Build history of the part. All positions in model axes, mm. Face numbers are marked on the shaded views. A direction names the side the tool comes from. Give positions to 0.01 mm unless a question says otherwise; leave off trailing zeros. Order: outer loops, then holes, each group sorted by start corner. A loop starts at its lowest first (then second) coordinate and runs counter-clockwise, first axis right, second up. Notation, with made-up numbers: (88, 70) -> (128, 70) arc R22 ccw to (128, 96) -> close; hole circle Ø2 at (31, 77). An arc over 180 degrees is marked (long way). One line per question, with ' | ' between items. Start each with the question number.
(1) Cut at A-A (y = 4). Give the cut face in (x, z) (3 decimals).
(2) Pin check, flat tips, straight feed: pin 1 Ø2.5 at (x, z) = (22.5, -14.5) entering from -Y (3 decimals); pin 2 Ø4 at (x, z) = (14, -29) entering from +Y (3 decimals); pin 3 Ø1.9 at (y, z) = (4, -10) entering from -X; pin 4 Ø1.5 at (x, z) = (-4, -19) entering from +Y. Stop position of each tip, or through.
(3) Drill centre lines: L1, parallel to X at y = 3.5, z = -11.43; L2, parallel to Z at x = 8, y = 2.25; L3, parallel to X at y = 1, z = -11.5. Where is each one in solid material? Low to high. Write a range as from..to.
(4) Which spindle directions (+Z, -Z, +X, -X, +Y, -Y) get a long thin tool onto all of the face, cutting with end or side? Do the marked faces 1, 2, 3 and 4. Say none if no direction does.
(5) Cut at C-C (z = -12.7). Give the cut face in (x, y) (3 decimals), then the cut area to 3 significant figures.
(6) Cut at D-D (y = 0.5). Give the cut face in (x, z) (3 decimals).
(7) Cut at B-B (x = 12.7). Give the cut face in (y, z) (3 decimals).
Autodesk Inventor part; units mm, degrees
ref_plane "YZ Plane" through (0, 0, 0) normal (1, 0, 0) x (0, 1, 0)
ref_plane "XZ Plane" through (0, 0, 0) normal (0, 1, 0) x (-1, 0, 0)
ref_plane "XY Plane" through (0, 0, 0) normal (0, 0, 1) x (1, 0, 0)
sketch "Sketch1" plane through (0, 0, 0) normal (0, 1, 0) x (-1, 0, 0)
  line L0 (0, 0) -> (-25.4, 0)
  line L1 (-25.4, 0) -> (-25.4, -25.4)
  line L2 (-25.4, -25.4) -> (0, -25.4)
  line L3 (0, -25.4) -> (0, 0)
  dimension "d0" = 25.4
extrude "Extrusion1" add sketch "Sketch1" along normal blind 6.35
sketch "Sketch2" plane through (0, 6.35, 0) normal (0, 1, 0) x (1, 0, 0)
  circle A0 centre (8.4667, 13.97) radius 0.635
  circle A1 centre (16.9333, 13.97) radius 0.635
  circle A2 centre (16.9333, 11.43) radius 0.635
  circle A3 centre (8.4667, 11.43) radius 0.635
  line L0 (25.4, 0) -> (25.4, 25.4)
  line L1 (0, 0) -> (25.4, 0)
  dimension "d3" = 8.4667
  dimension "d4" = 8.4667
  dimension "d5" = 2.54
  dimension "d6" = 1.27
  dimension "d7" = 11.43
extrude "Extrusion2" cut sketch "Sketch2" against normal blind 6.35
sketch "Sketch4" plane through (0, 0, 0) normal (0, -1, 0) x (1, 0, 0)
  line L0 (25.4, -25.4) -> (0, -25.4)
  arc A0 (9.525, -25.4) -> (15.875, -25.4) centre (12.7, -28.575) ccw
  line L1 (15.875, -25.4) -> (9.525, -25.4)
  point P0 (0, 0)
  dimension "d10" = 90
  dimension "d11" = 6.35
  dimension "d12" = 9.525
extrude "Extrusion3" add sketch "Sketch4" against normal blind 3.175
sketch "Sketch6" plane through (0, 0, 0) normal (0, -1, 0) x (1, 0, 0)
  line L0 (25.4, 0) -> (25.4, -25.4)
  arc A0 (25.4, -9.525) -> (25.4, -15.875) centre (22.225, -12.7) ccw
  line L1 (25.4, -15.875) -> (25.4, -9.525)
  point P0 (0, 0)
  dimension "d21" = 6.35
  dimension "d22" = 90
  dimension "d23" = 9.525
extrude "Extrusion5" cut sketch "Sketch6" against normal blind 3.175
sketch "Sketch7" plane through (0, 0, 0) normal (0, -1, 0) x (1, 0, 0)
  line L0 (0, -25.4) -> (0, 0)
  arc A0 (0, -9.525) -> (0, -15.875) centre (-3.175, -12.7) ccw
  line L1 (0, -15.875) -> (0, -9.525)
  dimension "d26" = 6.35
  dimension "d27" = 90
  dimension "d28" = 9.525
extrude "Extrusion6" add sketch "Sketch7" against normal blind 3.175
equation "\"d1\" = 0.25 * d0"
equation "\"d3\" = 0.333333 * d0"
equation "\"d4\" = d3"
equation "\"d8\" = 0.25 * d0"
equation "\"d11\" = 0.25 * d0"
equation "\"d12\" = 0.375 * d0"
equation "\"d13\" = 0.5 * d1"
equation "\"d21\" = 0.25 * d0"
equation "\"d23\" = 0.375 * d0"
equation "\"d24\" = 0.5 * d1"
equation "\"d26\" = 0.25 * d0"
equation "\"d28\" = 0.375 * d0"
equation "\"d29\" = 0.5 * d1"
properties part number "pieceBase"
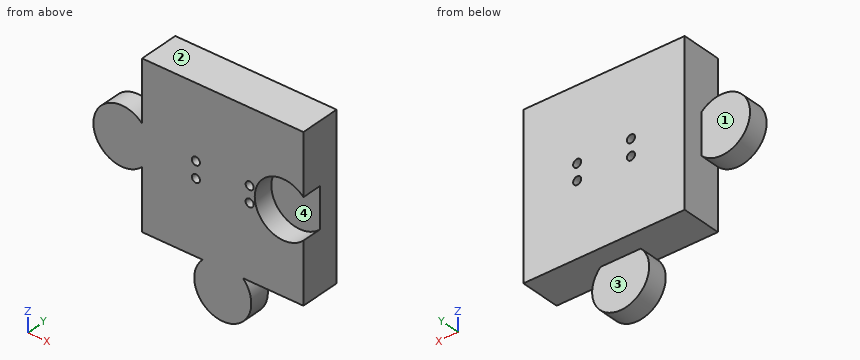
Result set:
1) outline: (0, -25.4) -> (25.4, -25.4) -> (25.4, 0) -> (0, 0) -> close; hole circle Ø1.27 at (8.467, -13.97); hole circle Ø1.27 at (8.467, -11.43); hole circle Ø1.27 at (16.933, -13.97); hole circle Ø1.27 at (16.933, -11.43)
2) pin 1: stops at y = 3.175 | pin 2: stops at y = 3.175 | pin 3: stops at x = -7.07 | pin 4: passes through
3) L1: x = 0..7.83, 9.1..16.3, 17.57..25.4 | L2: z = -25.4..-14.4, -13.54..-11.86, -11..0 | L3: x = -7.5..7.84, 9.1..16.3, 17.56..17.9
4) face 1: +Z, -Z, -X, +Y | face 2: +Z, +X, -X, +Y, -Y | face 3: -Z, +X, -X, +Y | face 4: -Y
5) outline: (-7.665, 0) -> (17.735, 0) -> (17.735, 3.175) -> (25.4, 3.175) -> (25.4, 6.35) -> (0, 6.35) -> (0, 3.175) -> (-7.665, 3.175) -> close | area: 161 mm2
6) outline: (0, -25.4) -> (9.525, -25.4) arc R4.49 ccw (long way) to (15.875, -25.4) -> (25.4, -25.4) -> (25.4, -15.875) arc R4.49 cw (long way) to (25.4, -9.525) -> (25.4, 0) -> (0, 0) -> (0, -9.525) arc R4.49 ccw (long way) to (0, -15.875) -> close; hole circle Ø1.27 at (8.467, -13.97); hole circle Ø1.27 at (8.467, -11.43); hole circle Ø1.27 at (16.933, -13.97); hole circle Ø1.27 at (16.933, -11.43)
7) outline: (0, -33.065) -> (3.175, -33.065) -> (3.175, -25.4) -> (6.35, -25.4) -> (6.35, 0) -> (0, 0) -> close
